Can you work these out from the model? Positions are in its coordinate system, mm. A direction names the side the tool comes from. Give positions to 0.01 mm unless a question says otherwise; leave off trailing zeros. Order: outer loops, then holes, each group sorted by start corner. A loop starts at its lowest first (then second) coordinate and runs counter-clockwise, first axis right, second up. Notation, with made-up numbers: M 12.5,40.5 L 54.5,40.5 A21 cw 54.5,73.5 Z; hole C -24,76 d7. An arc over 180 degrees is marked long. One line per question, with ' | ' between items. Start each with the question number.
1) If we section it at A-A, the plane x = 10.5: Please give me the cut outline in (y, z) (3 decimals), plus the area to 3 significant figures.
2) For faces 4 (the cylindrical face through (9.82, 8.77, 12.02)), 5 (the flat face through (26.251, 0, 8)), 6 (the flat face through (18, 9, 7.722)), 7 (the flat face through (35.662, 0, -18)), 8 (the flat face through (5, 0, 0)), which set-ups out of +Z, -Z, +X, -X, +Y, -Y let a thin tool reach every point of the face, with its end or its side?
3) Thinking about a two-plate mould opening in X: for faces 1 (the cylindrical face through (31.92, 0.01, -2.1)), 2 (the cylindrical face through (25.843, 8.774, 11.833)), 3 (the flat face through (9.411, 0, 8)), which applies, +X half, -X half, draft (parallel to the pull), parting line (faces both ways), or undercut?
4) I'm going to push flat-ended pins straight in: pin 1 Ø5 at (x, z) = (2.41, -33.2) entering from +Y (3 decimals); pin 2 Ø1.5 at (y, z) = (13.5, 7.5) entering from +X; pin 3 Ø8.5 at (x, y) = (19, 5) entering from -Z. Where does each tip first touch, or does it pass through?
5) If we section it at B-B, the plane y = 8.5: Please give me the cut outline in (x, z), plus the area to 3 significant figures.
6) If we section it at C-C, the plane z = 6: Please give me the cut outline in (x, y) (3 decimals), plus the area to 3 significant figures.
7) Please list where these lines run through material, in increasing order: line 1 along X through (y, z) = (0.5, -1.5); line 2 along Y through (x, z) = (24, -31) (3 decimals); line 3 along Z through (x, y) = (19, 11.25). Write a range as [from, to].
```python
from build123d import *

# Parameters (mm, degrees)
BOSS_EXTRUDE1_DEPTH = 0.635
BOSS_EXTRUDE2_DEPTH = 16.51
CUT_EXTRUDE2_REACH  = 55.289
SKETCH3_R           = 1.49987


with BuildPart() as part:
    # Sketch1 → Boss-Extrude1 (new, symmetric)
    with BuildSketch(Plane(origin=(0, 0, 0), x_dir=(1, 0, 0), z_dir=(0, 1, 0))):
        Polygon((0, 0), (9.4107, 0), (9.4107, -16.129), (26.2509, -16.129), (26.2509, 0), (35.6616, 0), (35.6616, 35.9918), (0, 35.9918), align=None)
    extrude(amount=BOSS_EXTRUDE1_DEPTH, both=True)

    # Sketch2 → Boss-Extrude2 (add)
    with BuildSketch(Plane(origin=(0, 0.635, 0), x_dir=(1, 0, 0), z_dir=(0, 1, 0))):
        with BuildLine():
            Line((14.0208, -7.7216), (21.6408, -7.7216))
            ThreePointArc((21.6408, -7.7216), (25.8445, -11.9253), (21.6408, -16.129))
            Line((21.6408, -16.129), (14.0208, -16.129))
            ThreePointArc((14.0208, -16.129), (9.8171, -11.9253), (14.0208, -7.7216))
        make_face()
    extrude(amount=BOSS_EXTRUDE2_DEPTH)

    # Sketch3 → Cut-Extrude2 (cut, up to next)
    with BuildSketch(Plane(origin=(0, 0.635, 0), x_dir=(1, 0, 0), z_dir=(0, 1, 0)), mode=Mode.PRIVATE) as cut_extrude2_sk1:
        with Locations(Location((2.413, 33.1978, 0), (0, 0, 270))):
            Circle(SKETCH3_R)
    cut_extrude2_tool1 = extrude(cut_extrude2_sk1.sketch, amount=-CUT_EXTRUDE2_REACH, mode=Mode.PRIVATE) & part.part
    # Sketch3 → Cut-Extrude2 (cut, up to next)
    with BuildSketch(Plane(origin=(0, 0.635, 0), x_dir=(1, 0, 0), z_dir=(0, 1, 0)), mode=Mode.PRIVATE) as cut_extrude2_sk2:
        with Locations(Location((2.413, 2.794, 0), (0, 0, 90))):
            Circle(SKETCH3_R)
    cut_extrude2_tool2 = extrude(cut_extrude2_sk2.sketch, amount=-CUT_EXTRUDE2_REACH, mode=Mode.PRIVATE) & part.part
    # Sketch3 → Cut-Extrude2 (cut, up to next)
    with BuildSketch(Plane(origin=(0, 0.635, 0), x_dir=(1, 0, 0), z_dir=(0, 1, 0)), mode=Mode.PRIVATE) as cut_extrude2_sk3:
        with Locations(Location((33.2486, 2.794, 0), (0, 0, 270))):
            Circle(SKETCH3_R)
    cut_extrude2_tool3 = extrude(cut_extrude2_sk3.sketch, amount=-CUT_EXTRUDE2_REACH, mode=Mode.PRIVATE) & part.part
    # Sketch3 → Cut-Extrude2 (cut, up to next)
    with BuildSketch(Plane(origin=(0, 0.635, 0), x_dir=(1, 0, 0), z_dir=(0, 1, 0)), mode=Mode.PRIVATE) as cut_extrude2_sk4:
        with Locations(Location((33.2486, 33.1978, 0), (0, 0, 90))):
            Circle(SKETCH3_R)
    cut_extrude2_tool4 = extrude(cut_extrude2_sk4.sketch, amount=-CUT_EXTRUDE2_REACH, mode=Mode.PRIVATE) & part.part
    add(cut_extrude2_tool1.solids().sort_by_distance((2.413, 0.635, -33.1978))[0], mode=Mode.SUBTRACT)
    add(cut_extrude2_tool2.solids().sort_by_distance((2.413, 0.635, -2.794))[0], mode=Mode.SUBTRACT)
    add(cut_extrude2_tool3.solids().sort_by_distance((33.2486, 0.635, -2.794))[0], mode=Mode.SUBTRACT)
    add(cut_extrude2_tool4.solids().sort_by_distance((33.2486, 0.635, -33.1978))[0], mode=Mode.SUBTRACT)


solid = part.part
```
Results found:
1) outline: M -0.635,-35.992 L 0.635,-35.992 L 0.635,9.629 L 17.145,9.629 L 17.145,14.222 L 0.635,14.222 L 0.635,16.129 L -0.635,16.129 Z | area: 142 mm²
2) face 4: -X, +Y | face 5: +Z, +X, +Y, -Y | face 6: -Z, +X, -X, +Y | face 7: +Z, -Z, +X, +Y, -Y | face 8: +Z, -X, +Y, -Y
3) face 1: undercut | face 2: +X half | face 3: -X half
4) pin 1: stops at y = 0.635 | pin 2: stops at x = 23.68 | pin 3: stops at z = 7.72
5) outline: M 14.02,7.72 L 21.64,7.72 A4.2 ccw 21.64,16.13 L 14.02,16.13 A4.2 ccw Z | area: 120 mm²
6) outline: M 9.411,-0.635 L 26.251,-0.635 L 26.251,0.635 L 9.411,0.635 Z | area: 21.4 mm²
7) line 1: x = [0, 1.65], [3.17, 32.49], [34.01, 35.66] | line 2: y = [-0.635, 0.635] | line 3: z = [7.72, 16.13]
